Part model, mm, in its own coordinate system. A direction names the side the tool comes from. Give positions to 0.01 mm unless a question says otherwise; leave off trailing zeros. Write each loop counter-clockwise with the first axis right and the second up, starting at its lowest first coordinate (ties: lowest second). Pieces come first, ordered by that corner, then holes.
```python
from build123d import *

# Parameters (mm, degrees)
SKETCH1_W           = 30
SKETCH1_H           = 36
BOSS_EXTRUDE1_DEPTH = 30
SKETCH3_R           = 12.375
CUT_EXTRUDE1_DEPTH  = 40
SKETCH5_R           = 1.875
CUT_EXTRUDE2_DEPTH  = 40
CUT_EXTRUDE3_START  = 15
SKETCH7_W           = 36
SKETCH7_H           = 15
CUT_EXTRUDE3_DEPTH  = 31
SKETCH8_R           = 5.75
BOSS_EXTRUDE2_DEPTH = 3.7
SKETCH11_R          = 2.92
CUT_EXTRUDE5_DEPTH  = 3.7
SKETCH12_R          = 1.75
CUT_EXTRUDE6_DEPTH  = 3.7
SKETCH14_R          = 2.55
CUT_EXTRUDE8_DEPTH  = 13.5


with BuildPart() as part:
    # Sketch1 → Boss-Extrude1 (new body)
    with BuildSketch(Plane(origin=(0, 0, 0), x_dir=(1, 0, 0), z_dir=(0, 1, 0))):
        Rectangle(SKETCH1_W, SKETCH1_H)
    extrude(amount=BOSS_EXTRUDE1_DEPTH)

    # Sketch3 → Cut-Extrude1 (cut)
    with BuildSketch(Plane(origin=(15, 0, 0), x_dir=(0, 0, -1), z_dir=(1, 0, 0))):
        with Locations((0, 15)):
            Circle(SKETCH3_R)
    extrude(amount=-CUT_EXTRUDE1_DEPTH, mode=Mode.SUBTRACT)

    # Sketch5 → Cut-Extrude2 (cut)
    with BuildSketch(Plane(origin=(0, 30, 0), x_dir=(1, 0, 0), z_dir=(0, 1, 0))):
        with Locations((-12.25, 15.25)):
            Circle(SKETCH5_R)
        with Locations((-12.25, -15.25)):
            Circle(SKETCH5_R)
        with Locations((12.25, -15.25)):
            Circle(SKETCH5_R)
        with Locations((12.25, 15.25)):
            Circle(SKETCH5_R)
    extrude(amount=-CUT_EXTRUDE2_DEPTH, mode=Mode.SUBTRACT)

    # Sketch7 → Cut-Extrude3 (cut, through all)
    with BuildSketch(Plane(origin=(0, 0, 0), x_dir=(0, 0, -1), z_dir=(1, 0, 0)).offset(CUT_EXTRUDE3_START)):
        with Locations((0, 7.5)):
            Rectangle(SKETCH7_W, SKETCH7_H)
    extrude(amount=-CUT_EXTRUDE3_DEPTH, mode=Mode.SUBTRACT)

    # Sketch8 → Boss-Extrude2 (add)
    with BuildSketch(Plane(origin=(0, 30, 0), x_dir=(1, 0, 0), z_dir=(0, 1, 0))):
        Circle(SKETCH8_R)
    extrude(amount=BOSS_EXTRUDE2_DEPTH)

    # Sketch11 → Cut-Extrude5 (cut)
    with BuildSketch(Plane(origin=(0, 33.7, 0), x_dir=(1, 0, 0), z_dir=(0, 1, 0))):
        Circle(SKETCH11_R)
    extrude(amount=-CUT_EXTRUDE5_DEPTH, mode=Mode.SUBTRACT)

    # Sketch12 → Cut-Extrude6 (cut)
    with BuildSketch(Plane(origin=(0, 30, 0), x_dir=(1, 0, 0), z_dir=(0, 1, 0))):
        Circle(SKETCH12_R)
    extrude(amount=-CUT_EXTRUDE6_DEPTH, mode=Mode.SUBTRACT)

    # Sketch14 → Cut-Extrude8 (cut)
    with BuildSketch(Plane.XZ.offset(-15)):
        Circle(SKETCH14_R)
    extrude(amount=-CUT_EXTRUDE8_DEPTH, mode=Mode.SUBTRACT)


solid = part.part
```
1) Saw through at D-D, the plane y = 20. Write the cut outline in (x, z) (3 decimals), then the cut area to 3 significant figures.
Answers follow:
outline: (-15, -18) - (15, -18) - (15, -11.32) - (-15, -11.32) - close; (-15, 11.32) - (15, 11.32) - (15, 18) - (-15, 18) - close; hole circle Ø3.75 at (-12.25, -15.25); hole circle Ø3.75 at (-12.25, 15.25); hole circle Ø3.75 at (12.25, -15.25); hole circle Ø3.75 at (12.25, 15.25)
area: 357 mm2
2) Pin check, flat tips, straight feed: pin 1 Ø1.8 at (x, z) = (1, -0.5) entering from +Y; pin 2 Ø4.5 at (x, z) = (0, 0) entering from -Y; pin 3 Ø1.5 at (x, z) = (0, -0.5) entering from -Y. Stop position of each tip, or through.
Answers follow:
pin 1: stops at y = 30
pin 2: stops at y = 28.5
pin 3: passes through
3) Wall check: L1, parallel to X at y = 25.25, z = 15.25 (3 decimals); L2, parallel to X at y = 29.05, z = 0; L3, parallel to Z at x = 0, y = 29.65. Give the ranges that are in metal, low to high.
Answers follow:
L1: x = -15 to -14.125, -10.375 to 10.375, 14.125 to 15
L2: x = -15 to -1.75, 1.75 to 15
L3: z = -18 to -1.75, 1.75 to 18
4) Saw through at A-A, the plane x = 0. Write the cut outline in (y, z) (3 decimals).
Answers follow:
outline: (15, -18) - (30, -18) - (30, -5.75) - (33.7, -5.75) - (33.7, -2.92) - (30, -2.92) - (30, -1.75) - (28.5, -1.75) - (28.5, -2.55) - (27.109, -2.55) arc R12.375 cw to (15, -12.375) - close; (15, 12.375) arc R12.375 cw to (27.109, 2.55) - (28.5, 2.55) - (28.5, 1.75) - (30, 1.75) - (30, 2.92) - (33.7, 2.92) - (33.7, 5.75) - (30, 5.75) - (30, 18) - (15, 18) - close
5) Saw through at B-B, the plane z = -15.25. Write the cut outline in (x, y) (3 decimals), then the cut area to 4 significant figures.
Answers follow:
outline: (-15, 15) - (-14.125, 15) - (-14.125, 30) - (-15, 30) - close; (-10.375, 15) - (10.375, 15) - (10.375, 30) - (-10.375, 30) - close; (14.125, 15) - (15, 15) - (15, 30) - (14.125, 30) - close
area: 337.5 mm2
6) 3-axis set-ups, long thin cutter, end or side, ignore diameter. For faces 1 (the face through (2.785, 31.876, -0.877)), 2 (the face through (0, 15, -15)), 3 (the face through (-2.024, 27.794, -1.552)): which of +Z, -Z, +X, -X, +Y, -Y reach the whole face in a straight line?
Answers follow:
face 1: +Y
face 2: +Z, -Z, +X, -X, -Y
face 3: -Y
7) Saw through at C-C, the plane x = -12.25. Write the cut outline in (y, z) (3 decimals), then the cut area to 3 significant figures.
Answers follow:
outline: (15, -18) - (30, -18) - (30, -17.125) - (15, -17.125) - close; (15, -13.375) - (30, -13.375) - (30, 13.375) - (15, 13.375) - (15, 12.375) arc R12.375 cw to (15, -12.375) - close; (15, 17.125) - (30, 17.125) - (30, 18) - (15, 18) - close
area: 187 mm2
8) Two-plate mould, pull along X, no slides. Class faces 4 (the face through (6, 30, 0)), 5 (the face through (0, 30, 2)), 6 (the face through (-0.75, 31.82, -5.7)): +X half, -X half, draft (parallel to the pull), parting line (faces both ways), or undercut.
Answers follow:
face 4: draft
face 5: undercut
face 6: parting line
